The drawing under review shows one solid part. Ordinate dimensions are in mm from its lowest x, y, z. Round coordinates to 2 decimals unless told otherwise and drop trailing zeros. Order: outer loops, then holes, each group sorted by start corner. A loop starts at its lowest first (then second) coordinate and runs counter-clockwise, first axis right, second up. Notation, with made-up numbers: M 61.25,19.5 L 76.25,19.5 A16 cw 76.25,33.5 Z; hole C 82,74.25 d9. An arc over 180 degrees is marked long. Write item = value, one per line. Start each with the question number.
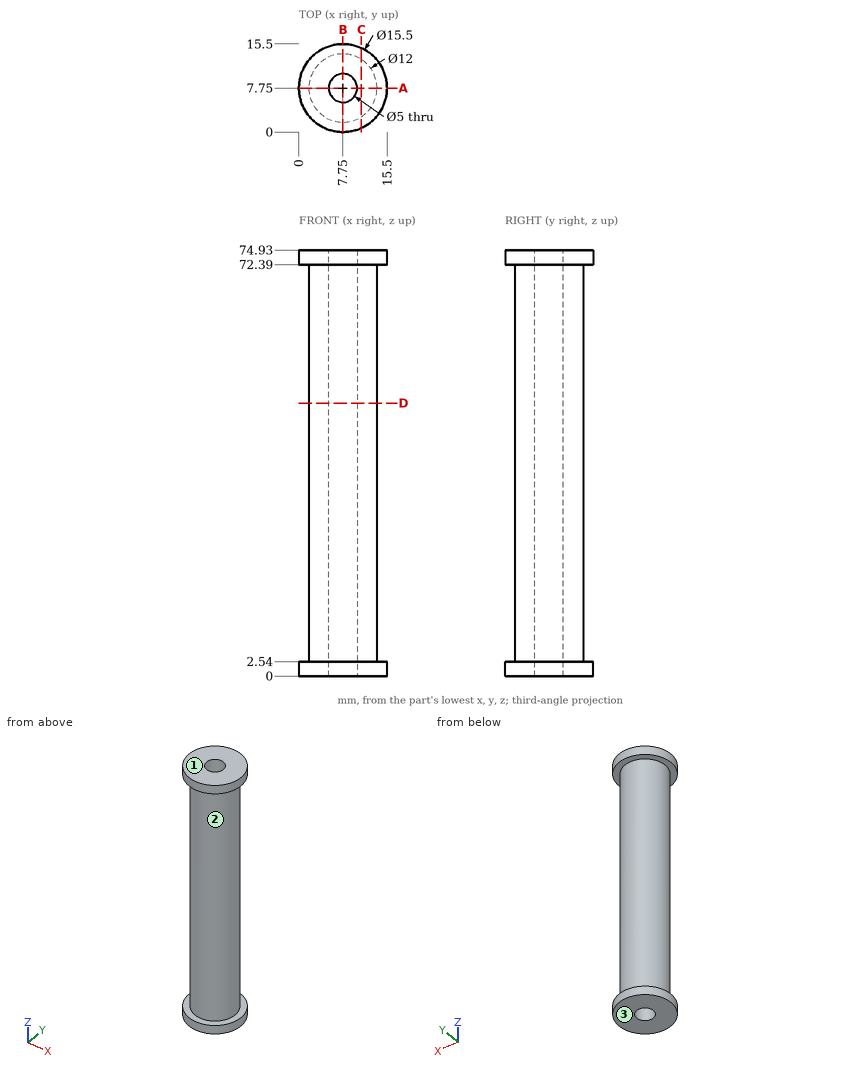
(1) Consider section A-A, the plane y = 7.75. Write out the cut boundary in (x, z).
(2) Consider section C-C, the plane x = 11. Write out the cut boundary in (y, z), then the cut area to 3 significant figures.
(3) Draft analysis for pull direction Z (two halves, no side actions). For the marked faces 1, 2 and 3, state which applies: pulls with the +Z half, pulls with the -Z half, needs draft (parallel to the pull), parting line crosses it, or undercut.
(4) Consider section D-D, the plane z = 48. Write out the cut boundary in (x, y), then the cut area to 3 significant figures.
(5) Insertion check: pin 1 (8 mm diameter, centred on x = 14, z = 46.5, fed in from +Y); pin 2 (5 mm diameter, centred on x = 9.5, z = 56.5, fed in from -Y); pin 3 (3 mm diameter, centred on x = 3.5, z = 20.5, fed in from -Y); pin 4 (4.5 mm diameter, centred on x = 7.75, y = 7.75, fed in from +Z). Each pin has a flat end and moves straight along its axis. Give the tip position at first contact, or say it passes through.
(6) For line 1 along Y through (x, z) = (7.75, 52.5); line 2 along Z through (x, y) = (10.25, 14.25); line 3 along X through (y, z) = (6.75, 69), list the stretches that pass through material, from the lowest coordinate up. Write a range as [from, to].
Completed:
q1.outline = M 0,0 L 5.25,0 L 5.25,74.93 L 0,74.93 L 0,72.39 L 1.75,72.39 L 1.75,2.54 L 0,2.54 Z; M 10.25,0 L 15.5,0 L 15.5,2.54 L 13.75,2.54 L 13.75,72.39 L 15.5,72.39 L 15.5,74.93 L 10.25,74.93 Z
q2.outline = M 0.71,0 L 14.79,0 L 14.79,2.54 L 12.79,2.54 L 12.79,72.39 L 14.79,72.39 L 14.79,74.93 L 0.71,74.93 L 0.71,72.39 L 2.71,72.39 L 2.71,2.54 L 0.71,2.54 Z
q2.area = 776 mm2
q3.face_1 = pulls with the +Z half
q3.face_2 = undercut
q3.face_3 = pulls with the -Z half
q4.outline = C 7.75,7.75 d12; hole C 7.75,7.75 d5
q4.area = 93.5 mm2
q5.pin_1 = 13.31
q5.pin_2 = 1.75
q5.pin_3 = 2.42
q5.pin_4 = through
q6.line_1 = [1.75, 5.25], [10.25, 13.75]
q6.line_2 = [0, 2.54], [72.39, 74.93]
q6.line_3 = [1.83, 5.46], [10.04, 13.67]
